from build123d import *

# Parameters (mm, degrees)
SALIENTE_EXTRUIR2_DEPTH = 3


with BuildPart() as part:
    # Croquis1 → Saliente-Extruir2 (new body)
    with BuildSketch(Plane.XY):
        with BuildLine():
            Line((-7.016617782, 12.62270249), (-10.016617782, 12.62270249))
            Line((-10.016617782, 12.62270249), (-10.016617782, 27.62270249))
            ThreePointArc((-10.016617782, 27.62270249), (-15.981083876, 22.223207554), (-24.016617782, 22.62270249))
            ThreePointArc((-24.016617782, 22.62270249), (-25.44554997, 16.172955022), (-31.016617782, 12.62270249))
            ThreePointArc((-31.016617782, 12.62270249), (-33.901410943, 6.263831835), (-38.016617782, 0.62270249))
            ThreePointArc((-38.016617782, 0.62270249), (-36.124451454, -6.87729751), (-38.016617782, -14.37729751))
            ThreePointArc((-38.016617782, -14.37729751), (-28.016617782, -10.235161886), (-18.016617782, -14.37729751))
            Line((-18.016617782, -14.37729751), (-10.016617782, -2.37729751))
            Line((-10.016617782, -2.37729751), (-7.016617782, -2.37729751))
            Line((-7.016617782, -2.37729751), (0.983382218, -14.37729751))
            ThreePointArc((0.983382218, -14.37729751), (10.983382218, -10.235161886), (20.983382218, -14.37729751))
            ThreePointArc((20.983382218, -14.37729751), (19.09121589, -6.87729751), (20.983382218, 0.62270249))
            ThreePointArc((20.983382218, 0.62270249), (16.868175379, 6.263831835), (13.983382218, 12.62270249))
            ThreePointArc((13.983382218, 12.62270249), (8.412314406, 16.172955022), (6.983382218, 22.62270249))
            ThreePointArc((6.983382218, 22.62270249), (-1.052151688, 22.223207554), (-7.016617782, 27.62270249))
            Line((-7.016617782, 27.62270249), (-7.016617782, 12.62270249))
        make_face()
    extrude(amount=SALIENTE_EXTRUIR2_DEPTH)


solid = part.part
Can you work these out from the model? Positions are in its coordinate system, mm. A direction names the side the tool comes from. Coordinates: 2 decimals unless noted, no trailing zeros. Write each loop counter-clockwise with the first axis right and the second up, starting at its lowest first coordinate (ties: lowest second). Pieces come first, ordered by that corner, then holes. Notation, with made-up numbers: (32, 34) -> (72, 34) arc R24 cw to (72, 60) -> close; hole circle Ø9 at (-0.75, 47.5). An arc over 180 degrees is marked (long way). Answer as CSV lines item,"result".
1) If we mould it in two halves opening along Y, with no side actions, what happens to faces 4 (the flat face through (-9, -2.377, 1)), 5 (the cylindrical face through (-36.125, -6.768, 1.479)), 6 (the flat face through (-7.017, 20, 1)), 7 (the cylindrical face through (8.467, 16.096, 1.479))? For each: +Y half, -Y half, draft (parallel to the pull), parting line (faces both ways), or undercut.
Check result:
face 4,"-Y half"
face 5,"undercut"
face 6,"draft"
face 7,"undercut"
2) If we section it at D-D on y = 7: Please give me the cut outline in (x, z).
Check result:
outline,"(-33.48, 0) -> (16.45, 0) -> (16.45, 3) -> (-33.48, 3) -> close"
3) If we section it at A-A on y = -6: Please give me the cut outline in (x, z).
Check result:
outline,"(-36.15, 0) -> (-12.43, 0) -> (-12.43, 3) -> (-36.15, 3) -> close; (-4.6, 0) -> (19.12, 0) -> (19.12, 3) -> (-4.6, 3) -> close"
4) Will these pins go through, and if not, where does the flat tip stop? P1, Ø12, axis at x = -8, y = -6, coming from the -Z side; P2, Ø1, axis at x = -12.5, z = 0.5, coming from the -Y side; P3, Ø0.9, axis at x = -8, z = 1.5, coming from the +Y side; P4, Ø6, axis at x = -28.5, y = 23.5, coming from the +Z side.
Check result:
P1,"z = 0"
P2,"y = -6.85"
P3,"y = 12.62"
P4,"through"
5) If I drill on line 1 (X direction, y = -7, z = 0.95); line 2 (X direction, y = 16, z = 0.95); line 3 (Y direction, x = 5.5, z = 2.5), over which ranges is the centre line in solid material (lowest first)? Write a range as from..to.
Check result:
line 1,"-36.12..-13.1, -3.93..19.09"
line 2,"-25.57..-10.02, -7.02..8.54"
line 3,"-11.34..22.05"
6) If we section it at B-B on z = 0.8: Please give me the cut outline in (x, y), then the cut area to 3 significant figures.
Check result:
outline,"(-38.02, -14.38) arc R14.14 cw to (-18.02, -14.38) -> (-10.02, -2.38) -> (-7.02, -2.38) -> (0.98, -14.38) arc R14.14 cw to (20.98, -14.38) arc R15.81 cw to (20.98, 0.62) arc R34.23 cw to (13.98, 12.62) arc R8.63 cw to (6.98, 22.62) arc R10.51 cw to (-7.02, 27.62) -> (-7.02, 12.62) -> (-10.02, 12.62) -> (-10.02, 27.62) arc R10.51 cw to (-24.02, 22.62) arc R8.63 cw to (-31.02, 12.62) arc R34.23 cw to (-38.02, 0.62) arc R15.81 cw to start"
area,"1,530 mm²"
7) On a 3-axis mill with a long thin cutter (end or side, diameter ignored), from which of +Z, -Z, +X, -X, +Y, -Y can I reach the whole of each face in a straight line? I mean faces 1 (the flat face through (-14.1, -8.5, 1.5)), 2 (the flat face through (-8, 12.623, 1)), 3 (the cylindrical face through (-33.85, 6.35, 1.48)). Say none if no direction works.
Check result:
face 1,"+Z, -Z, -Y"
face 2,"+Z, -Z, +Y"
face 3,"+Z, -Z, -X, +Y"
8) If we section it at C-C on x = -3.5: Please give me the cut outline in (y, z).
Check result:
outline,"(-7.65, 0) -> (23.48, 0) -> (23.48, 3) -> (-7.65, 3) -> close"
